Autodesk Inventor part; units mm, degrees
ref_plane "ABDECKPROFIL_XY" through (0, 0, 287) normal (0, 0, -1) x (1, 0, 0)
ref_plane "ABDECKPROFIL_YZ" through (0, 0, 287) normal (1, 0, 0) x (0, -1, 0)
ref_plane "ABDECKPROFIL_ZX" through (0, 0, 287) normal (0, -1, 0) x (0, 0, -1)
sketch "Sketch_1" plane through (0, 0, 0) normal (0, 0, 1) x (1, 0, 0)
  line L0 (-6.5, -6.2) -> (-5, -7.8)
  line L1 (-5, -7.8) -> (-3.226, -1.1793)
  arc A0 (-3.0947, -1.0409) -> (-3.226, -1.1793) centre (-3.0328, -1.2311) ccw
  arc A1 (3.0947, -1.0409) -> (-3.0947, -1.0409) centre (0, -10.55) ccw
  arc A2 (3.226, -1.1793) -> (3.0947, -1.0409) centre (3.0328, -1.2311) ccw
  line L2 (3.226, -1.1793) -> (5, -7.8)
  line L3 (5, -7.8) -> (6.5, -6.2)
  line L4 (6.5, -6.2) -> (5.326, -5.9257)
  line L5 (5.326, -5.9257) -> (4.9136, -4.3864)
  line L6 (4.9136, -4.3864) -> (5.5, -3.8)
  line L7 (5.5, -3.8) -> (4.4843, -2.7843)
  line L8 (4.4843, -2.7843) -> (4.0598, -1.2)
  line L9 (4.0598, -1.2) -> (5.8, -1.2)
  arc A3 (5.8, -1.2) -> (6, -1) centre (5.8, -1) ccw
  line L10 (6, -1) -> (6, -0.2)
  arc A4 (6, -0.2) -> (5.8, 0) centre (5.8, -0.2) ccw
  line L11 (5.8, 0) -> (-5.8, 0)
  arc A5 (-5.8, 0) -> (-6, -0.2) centre (-5.8, -0.2) ccw
  line L12 (-6, -0.2) -> (-6, -1)
  arc A6 (-6, -1) -> (-5.8, -1.2) centre (-5.8, -1) ccw
  line L13 (-5.8, -1.2) -> (-4.0598, -1.2)
  line L14 (-4.0598, -1.2) -> (-4.4843, -2.7843)
  line L15 (-4.4843, -2.7843) -> (-5.5, -3.8)
  line L16 (-5.5, -3.8) -> (-4.9136, -4.3864)
  line L17 (-4.9136, -4.3864) -> (-5.326, -5.9257)
  line L18 (-5.326, -5.9257) -> (-6.5, -6.2)
extrude "Extrusion1" add sketch "Sketch_1" along normal blind 287
ref_plane "ABDECKPROFIL_XY" through (0, 0, 287) normal (0, 0, -1) x (1, 0, 0)
ref_plane "ABDECKPROFIL_YZ" through (0, 0, 287) normal (1, 0, 0) x (0, -1, 0)
ref_plane "ABDECKPROFIL_ZX" through (0, 0, 287) normal (0, -1, 0) x (0, 0, -1)
properties part number "SLZ_63_Abdeck_Profil#_2871"
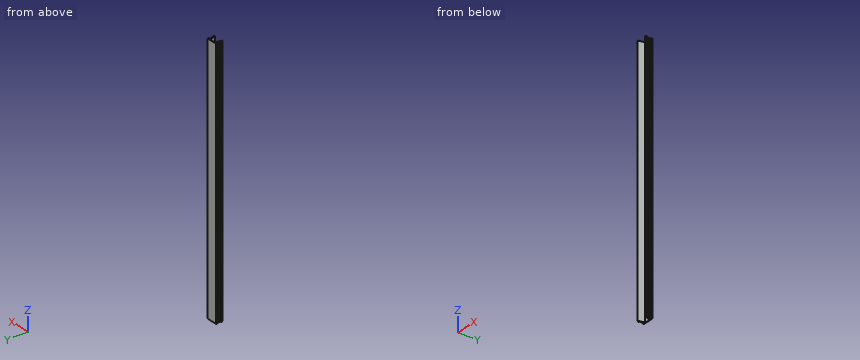
Here's how the part is built. I have some questions about the finished solid (model axes, mm). Coordinates: 2 decimals unless noted, no trailing zeros. Loops run counter-clockwise (first coordinate to the right, second up) from the corner with the lowest first, then second, coordinate; pieces in that order, holes last.
1. I need wall thicknesses on L1, parallel to X at y = -4.5, z = 258; L2, parallel to X at y = -7.5, z = 141.5; L3, parallel to Y at x = 3, z = 31.5. Which ranges of each line are inside material? Lowest first, please.
2. For P1, Ø4, axis at y = -5.5, z = 33.5, coming from the -X side; P2, Ø1.4, axis at x = 5, z = 145, coming from the -Y side, each with a flat end and sliding along its axis, tell me the tip position at first contact or that it passes through.
3. Imagine slicing it at B-B, the plane x = -0.75. Please give me the cut outline in (y, z), and give its area (3 significant figures).
4. Imagine slicing it at A-A, the plane z = 259.5. Please give me the cut outline in (x, y).
Taken from the geometry:
1. L1: x = -4.94 to -4.12, 4.12 to 4.94
1. L2: x = -5.28 to -4.92, 4.92 to 5.28
1. L3: y = -1.01 to 0
2. P1: stops at x = -6.5
2. P2: stops at y = -7.8
3. outline: (-0.58, 0) - (0, 0) - (0, 287) - (-0.58, 287) - close
3. area: 166 mm2
4. outline: (-6.5, -6.2) - (-5, -7.8) - (-3.23, -1.18) arc R0.2 cw to (-3.09, -1.04) arc R10 cw to (3.09, -1.04) arc R0.2 cw to (3.23, -1.18) - (5, -7.8) - (6.5, -6.2) - (5.33, -5.93) - (4.91, -4.39) - (5.5, -3.8) - (4.48, -2.78) - (4.06, -1.2) - (5.8, -1.2) arc R0.2 ccw to (6, -1) - (6, -0.2) arc R0.2 ccw to (5.8, 0) - (-5.8, 0) arc R0.2 ccw to (-6, -0.2) - (-6, -1) arc R0.2 ccw to (-5.8, -1.2) - (-4.06, -1.2) - (-4.48, -2.78) - (-5.5, -3.8) - (-4.91, -4.39) - (-5.33, -5.93) - close
